Geometry: final body of the model. Coordinates: model frame, mm. A direction names the side the tool comes from. Give positions to 0.01 mm unless a question says otherwise; leave off trailing zeros. Loops run counter-clockwise (first coordinate to the right, second up) from the corner with the lowest first, then second, coordinate; pieces in that order, holes last.
Autodesk Inventor part; units mm, degrees
ref_plane "YZ Plane" through (0, 0, 0) normal (1, 0, 0) x (0, 1, 0)
ref_plane "XZ Plane" through (0, 0, 0) normal (0, 1, 0) x (-1, 0, 0)
ref_plane "XY Plane" through (0, 0, 0) normal (0, 0, 1) x (1, 0, 0)
sketch "Szkic1" plane through (0, 0, 0) normal (0, 1, 0) x (-1, 0, 0)
  arc A0 (48.2455, -77.7225) -> (63.1896, -66.1474) centre (54.9934, -71) ccw
  arc A1 (46.3327, -79.628) -> (65.5129, -64.7719) centre (54.9934, -71) ccw
  arc A2 (17.7907, 10.5331) -> (-14.647, -14.5918) centre (0, 0) ccw
  arc A3 (20.1141, 11.9086) -> (-16.5598, -16.4974) centre (0, 0) ccw
  line L0 (65.5129, -64.7719) -> (20.1141, 11.9086)
  line L1 (46.3327, -79.628) -> (-16.5598, -16.4974)
  line L2 (17.7907, 10.5331) -> (63.1896, -66.1474)
  line L3 (48.2455, -77.7225) -> (-14.647, -14.5918)
  point P0 (0, 0)
extrude "Wyciągnięcie proste1" add sketch "Szkic1" along normal blind 10
properties part number "Pas zębaty 10 T5-295"
Item 1: Section query A-A on y = 5.75. Return loops of the section in (x, z) (1 decimal), plus the area to 3 significant figures.
Values follow:
outline: (-65.5, -64.8) arc R12.2 ccw to (-46.3, -79.6) - (16.6, -16.5) arc R23.4 ccw (long way) to (-20.1, 11.9) - close; hole (-63.2, -66.1) arc R9.5 ccw to (-48.2, -77.7) - (14.6, -14.6) arc R20.7 ccw (long way) to (-17.8, 10.5) - close
area: 768 mm2
Item 2: Section query B-B on x = -13. Return loops of the section in (y, z), plus the area to 3 significant figures.
Values follow:
outline: (0, -46.17) - (10, -46.17) - (10, -42.34) - (0, -42.34) - close; (0, 16.08) - (10, 16.08) - (10, 19.43) - (0, 19.43) - close
area: 71.8 mm2
Item 3: Section query C-C on z = -2.5. Return loops of the section in (x, y).
Values follow:
outline: (-28.64, 0) - (-25.51, 0) - (-25.51, 10) - (-28.64, 10) - close; (20.52, 0) - (23.24, 0) - (23.24, 10) - (20.52, 10) - close
Item 4: Draft query along Z for faces 1 (the face through (13.045, 4.93, 16.04)), 2 (the face through (14.748, 4.93, 18.135)), 3 (the face through (-35, 0, -18)), 4 (the face through (-15.327, 4.93, -48.505)). Return one class per face: +Z half, -Z half, draft (parallel to the pull), parting line (faces both ways), or undercut.
Values follow:
face 1: undercut
face 2: parting line
face 3: draft
face 4: -Z half
Item 5: Set-up query: faces 5 (the face through (-43.13, 4.93, -26.97)), 6 (the face through (-40.17, 4.93, -27.27)). Return all of +Z, -Z, +X, -X, +Y, -Y with unobstructed straight access to the full face (end or side cutting, diameter ignored); none if empty.
Values follow:
face 5: +Z, -X, +Y, -Y
face 6: +Y, -Y
Item 6: Pin query (flat end, axial travel): pin 1 (5 mm diameter, centred on x = 6.5, y = 2, fed in from -Z); pin 2 (1.5 mm diameter, centred on x = -57, y = 6, fed in from -Z); pin 3 (1.5 mm diameter, centred on y = 6, z = -40.5, fed in from +X). Return the tip coordinate at first contact, or that it passes through.
Values follow:
pin 1: stops at z = -29.1
pin 2: stops at z = -83.16
pin 3: stops at x = -6.61
Item 7: Ray query, probe 1 along X at (y, z) = (6.5, -45.5); probe 2 along X at (y, z) = (5.75, -71); probe 3 along Z at (x, y) = (-58, 8.5). Return the intervals inside material, ascending.
Values follow:
probe 1: x = -54.1 to -50.97, -16.14 to -12.33
probe 2: x = -67.22 to -64.52, -41.55 to -37.74
probe 3: z = -82.85 to -80.04, -57.38 to -52.08
